The model under review builds one solid part; all positions refer to its coordinate system, in mm. A direction names the side the tool comes from. Give positions to 0.01 mm unless a question says otherwise; leave off trailing zeros. Write each loop counter-clockwise with the first axis right and the second up, starting at its lowest first coordinate (ties: lowest second). Pieces come first, ordered by that corner, then holes. Notation, with made-up numbers: (-19.5, 16) - (17.5, 16) arc R14 cw to (17.5, 41) - close; hole circle Ø3 at (-8.75, 78.5). An arc over 180 degrees is marked (long way). Write item = value, one per line.
```python
from build123d import *

# Parameters (mm, degrees)
BOSS_EXTRUDE1_DEPTH      = 23.8125
BOSS_EXTRUDE1_DEPTH_BACK = 23.8125
CUT_EXTRUDE1_DEPTH       = 58.710288262
CUT_EXTRUDE1_DEPTH_BACK  = 58.710288262
SKETCH6_R                = 3.5687
CUT_EXTRUDE2_DEPTH       = 58.710288262
SKETCH7_R                = 3.5687
CUT_EXTRUDE3_DEPTH       = 58.710288262


with BuildPart() as part:
    # Sketch4 → Boss-Extrude1 (new, two sides: drawn at the far end of the back side and taken through both)
    with BuildSketch(Plane.XY.offset(-BOSS_EXTRUDE1_DEPTH_BACK)):
        with BuildLine():
            Line((-25.4, 25.4), (-25.4, -25.4))
            Line((-25.4, -25.4), (25.4, -25.4))
            ThreePointArc((25.4, -25.4), (24.001376302, -22.023423698), (20.6248, -20.6248))
            Line((20.6248, -20.6248), (-17.4498, -20.6248))
            ThreePointArc((-17.4498, -20.6248), (-19.69486403, -19.69486403), (-20.6248, -17.4498))
            Line((-20.6248, -17.4498), (-20.6248, 20.6248))
            ThreePointArc((-20.6248, 20.6248), (-22.023423698, 24.001376302), (-25.4, 25.4))
        make_face()
    extrude(amount=BOSS_EXTRUDE1_DEPTH + BOSS_EXTRUDE1_DEPTH_BACK)

    # Sketch5 → Cut-Extrude1 (cut, two sides: drawn at the far end of the back side and taken through both)
    with BuildSketch(Plane(origin=(-20.6248, 0, 0), x_dir=(0, 0, -1), z_dir=(1, 0, 0)).offset(-CUT_EXTRUDE1_DEPTH_BACK)):
        Polygon((23.8125, 25.4), (0, 25.4), (23.8125, -17.4498), align=None)
    extrude(amount=CUT_EXTRUDE1_DEPTH + CUT_EXTRUDE1_DEPTH_BACK, mode=Mode.SUBTRACT)

    # Sketch6 → Cut-Extrude2 (cut, through all)
    with BuildSketch(Plane(origin=(-20.6248, 0, 0), x_dir=(0, 0, -1), z_dir=(1, 0, 0))):
        with Locations(Location((-11.90625, 12.7, 0), (0, 0, 90))):
            Circle(SKETCH6_R)
        with Locations(Location((-11.90625, -12.7, 0), (0, 0, 270))):
            Circle(SKETCH6_R)
    extrude(amount=-CUT_EXTRUDE2_DEPTH, mode=Mode.SUBTRACT)

    # Sketch7 → Cut-Extrude3 (cut, through all)
    with BuildSketch(Plane(origin=(0, -20.6248, 0), x_dir=(1, 0, 0), z_dir=(0, 1, 0))):
        with Locations(Location((-12.7, 12.7, 0), (0, 0, 180))):
            Circle(SKETCH7_R)
        with Locations(Location((12.7, 12.7, 0), (0, 0, 180))):
            Circle(SKETCH7_R)
        with Locations((12.7, -12.7)):
            Circle(SKETCH7_R)
        with Locations((-12.7, -12.7)):
            Circle(SKETCH7_R)
    extrude(amount=-CUT_EXTRUDE3_DEPTH, mode=Mode.SUBTRACT)


solid = part.part
```
1. Take a section at D-D on z = 12.7. Give the boundary of the cut face in (x, y) (3 decimals), and give its area (3 significant figures).
Findings below:
outline = (-25.4, -25.4) - (-16.269, -25.4) - (-16.269, -20.625) - (-17.45, -20.625) arc R3.175 cw to (-20.625, -17.45) - (-20.625, -16.179) - (-25.4, -16.179) - close; (-25.4, -9.221) - (-20.625, -9.221) - (-20.625, 9.221) - (-25.4, 9.221) - close; (-25.4, 16.179) - (-20.625, 16.179) - (-20.625, 20.625) arc R4.775 ccw to (-25.4, 25.4) - close; (-9.131, -25.4) - (9.131, -25.4) - (9.131, -20.625) - (-9.131, -20.625) - close; (16.269, -25.4) - (25.4, -25.4) arc R4.775 ccw to (20.625, -20.625) - (16.269, -20.625) - close
area = 320 mm²
2. Machinability: for faces 1 (the flat face through (-20.625, 1, 5)), 2 (the flat face through (0, -25.4, 0)), which of the approach directions +Z, -Z, +X, -X, +Y, -Y give a long, thin tool a straight path to every point of the face, cutting with its end or side? Answer none if there is none.
Findings below:
face_1 = +Z, -Z, +X, +Y
face_2 = +Z, -Z, +X, -X, -Y
3. Take a section at B-B on z = -12.7. Give the boundary of the cut face in (x, y) (3 decimals), and give its area (3 significant figures).
Findings below:
outline = (-25.4, -25.4) - (-16.269, -25.4) - (-16.269, -20.625) - (-17.45, -20.625) arc R3.175 cw to (-20.625, -17.45) - (-20.625, 2.547) - (-25.4, 2.547) - close; (-9.131, -25.4) - (9.131, -25.4) - (9.131, -20.625) - (-9.131, -20.625) - close; (16.269, -25.4) - (25.4, -25.4) arc R4.775 ccw to (20.625, -20.625) - (16.269, -20.625) - close
area = 282 mm²
4. Take a section at C-C on y = -12.7. Give the boundary of the cut face in (x, z).
Findings below:
outline = (-25.4, -21.17) - (-20.62, -21.17) - (-20.62, 8.34) - (-25.4, 8.34) - close; (-25.4, 15.47) - (-20.62, 15.47) - (-20.62, 23.81) - (-25.4, 23.81) - close
5. Draft analysis for pull direction Y (two halves, no side actions). For faces 3 (the cylindrical face through (16.265, -22.979, -12.543)), 4 (the flat face through (-23.046, 4.275, -11.74)), 5 (the cylindrical face through (-22.98, 9.87, 9.73)), 6 (the cylindrical face through (-22.98, -9.87, 14.08)), state which applies: +Y half, -Y half, draft (parallel to the pull), parting line (faces both ways), or undercut.
Findings below:
face_3 = draft
face_4 = +Y half
face_5 = undercut
face_6 = undercut
6. Take a section at A-A on x = 12.7. Give the boundary of the cut face in (y, z).
Findings below:
outline = (-25.4, -23.81) - (-20.62, -23.81) - (-20.62, -16.27) - (-25.4, -16.27) - close; (-25.4, -9.13) - (-20.62, -9.13) - (-20.62, 9.13) - (-25.4, 9.13) - close; (-25.4, 16.27) - (-20.62, 16.27) - (-20.62, 23.81) - (-25.4, 23.81) - close
7. Insertion check: P1, Ø8, axis at x = -12.7, z = -12.7, coming from the +Y side; P2, Ø2, axis at y = 15, z = 3.5, coming from the +X side; P3, Ø11.5, axis at y = 12.7, z = 11.91, coming from the -X side. Each pin has a flat end and moves straight along its axis. Give the tip position at first contact, or say it passes through.
Findings below:
P1 = -20.62
P2 = -20.62
P3 = -25.4
8. For line 1 (Z direction, x = 12.7, y = -24.05); line 2 (Z direction, x = -12, y = -22); line 3 (Y direction, x = 5, z = 1), list the stretches that pass through material, from the lowest coordinate up. Write a range as from..to.
Findings below:
line_1 = -23.81..-16.27, -9.13..9.13, 16.27..23.81
line_2 = -23.81..-16.2, -9.2..9.2, 16.2..23.81
line_3 = -25.4..-20.62
